Verification items for the finished model (mm, model axes). A direction names the side the tool comes from. Round coordinates to 2 decimals unless told otherwise and drop trailing zeros. Write each loop counter-clockwise with the first axis right and the second up, starting at its lowest first coordinate (ties: lowest second). Pieces come first, ordered by that corner, then holes. Notation, with made-up numbers: (82.25, 44) - (98.25, 44) arc R23 cw to (98.25, 55) - close; hole circle Ø1 at (23, 61.25). An arc over 180 degrees is marked (long way). Answer as a JSON object with one key per item and string values.
```python
from build123d import *

# Parameters (mm, degrees)
F1_R     = 22.710134
F2_DEPTH = 25


with BuildPart() as f2:
    # F1 (on Top) → F2 (new body)
    with BuildSketch(Plane.XY):
        with BuildLine():
            Line((3.498161, 48.480518), (0, 48.958581))
            Line((0, 48.958581), (-3.498161, 48.480518))
            Line((-3.498161, 48.480518), (-5.9562, 36.306892))
            ThreePointArc((-5.9562, 36.306892), (-11.369418, 34.991471), (-16.521988, 32.873859))
            Line((-16.521988, 32.873859), (-25.666062, 41.277731))
            Line((-25.666062, 41.277731), (-28.777132, 39.608324))
            Line((-28.777132, 39.608324), (-31.326205, 37.165396))
            Line((-31.326205, 37.165396), (-26.159323, 25.871926))
            ThreePointArc((-26.159323, 25.871926), (-29.765523, 21.625918), (-32.689339, 16.88413))
            Line((-32.689339, 16.88413), (-45.026722, 18.308253))
            Line((-45.026722, 18.308253), (-46.562377, 15.129034))
            Line((-46.562377, 15.129034), (-47.188704, 11.654355))
            Line((-47.188704, 11.654355), (-36.370473, 5.554763))
            ThreePointArc((-36.370473, 5.554763), (-36.79221, 0), (-36.370473, -5.554763))
            Line((-36.370473, -5.554763), (-47.188704, -11.654355))
            Line((-47.188704, -11.654355), (-46.562377, -15.129034))
            Line((-46.562377, -15.129034), (-45.026722, -18.308253))
            Line((-45.026722, -18.308253), (-32.689339, -16.88413))
            ThreePointArc((-32.689339, -16.88413), (-29.765523, -21.625918), (-26.159323, -25.871926))
            Line((-26.159323, -25.871926), (-31.326205, -37.165396))
            Line((-31.326205, -37.165396), (-28.777132, -39.608324))
            Line((-28.777132, -39.608324), (-25.666062, -41.277731))
            Line((-25.666062, -41.277731), (-16.521988, -32.873859))
            ThreePointArc((-16.521988, -32.873859), (-11.369418, -34.991471), (-5.9562, -36.306892))
            Line((-5.9562, -36.306892), (-3.498161, -48.480518))
            Line((-3.498161, -48.480518), (0, -48.958581))
            Line((0, -48.958581), (3.498161, -48.480518))
            Line((3.498161, -48.480518), (5.9562, -36.306892))
            ThreePointArc((5.9562, -36.306892), (11.369418, -34.991471), (16.521988, -32.873859))
            Line((16.521988, -32.873859), (25.666062, -41.277731))
            Line((25.666062, -41.277731), (28.777132, -39.608324))
            Line((28.777132, -39.608324), (31.326205, -37.165396))
            Line((31.326205, -37.165396), (26.159323, -25.871926))
            ThreePointArc((26.159323, -25.871926), (29.765523, -21.625918), (32.689339, -16.88413))
            Line((32.689339, -16.88413), (45.026722, -18.308253))
            Line((45.026722, -18.308253), (46.562377, -15.129034))
            Line((46.562377, -15.129034), (47.188704, -11.654355))
            Line((47.188704, -11.654355), (36.370473, -5.554763))
            ThreePointArc((36.370473, -5.554763), (36.79221, 0), (36.370473, 5.554763))
            Line((36.370473, 5.554763), (47.188704, 11.654355))
            Line((47.188704, 11.654355), (46.562377, 15.129034))
            Line((46.562377, 15.129034), (45.026722, 18.308253))
            Line((45.026722, 18.308253), (32.689339, 16.88413))
            ThreePointArc((32.689339, 16.88413), (29.765523, 21.625918), (26.159323, 25.871926))
            Line((26.159323, 25.871926), (31.326205, 37.165396))
            Line((31.326205, 37.165396), (28.777132, 39.608324))
            Line((28.777132, 39.608324), (25.666062, 41.277731))
            Line((25.666062, 41.277731), (16.521988, 32.873859))
            ThreePointArc((16.521988, 32.873859), (11.369418, 34.991471), (5.9562, 36.306892))
            Line((5.9562, 36.306892), (3.498161, 48.480518))
        make_face()
        Circle(F1_R, mode=Mode.SUBTRACT)
    extrude(amount=F2_DEPTH)


solid = f2.part
```
1. Cross-section at B-B (x = 15). Record the boundary of the cut face in (y, z), plus the area to 3 significant figures.
Completed:
{"outline": "(-33.6, 0) - (-17.05, 0) - (-17.05, 25) - (-33.6, 25) - close; (17.05, 0) - (33.6, 0) - (33.6, 25) - (17.05, 25) - close", "area": "827 mm^2"}
2. Go/stop test with flat-tipped pins: pin 1 (1 mm diameter, centred on x = 37, z = 16, fed in from -Y); pin 2 (1 mm diameter, centred on x = -7, y = 25, fed in from -Z); pin 3 (10 mm diameter, centred on x = -13.5, z = 4, fed in from -Y); pin 4 (4 mm diameter, centred on y = 24, z = 6, fed in from +X). Record where each tip stops, or that it passes through.
Completed:
{"pin 1": "stops at y = -17.44", "pin 2": "stops at z = 0", "pin 3": "stops at y = -35.8", "pin 4": "stops at x = 29.49"}
3. Cross-section at C-C (y = 28.5). Record the boundary of the cut face in (x, z), plus the area to 3 significant figures.
Completed:
{"outline": "(-27.36, 0) - (27.36, 0) - (27.36, 25) - (-27.36, 25) - close", "area": "1,370 mm^2"}
4. Cross-section at A-A (y = 0). Record the boundary of the cut face in (x, z), plus the area to 3 significant figures.
Completed:
{"outline": "(-36.79, 0) - (-22.71, 0) - (-22.71, 25) - (-36.79, 25) - close; (22.71, 0) - (36.79, 0) - (36.79, 25) - (22.71, 25) - close", "area": "704 mm^2"}
5. Mould release check, pull along X, two halves, no side actions. Record for faces 1 (the face through (-46.88, -13.37, 12.32)), 2 (the face through (11.295, -35.016, 12.325)), 3 (the face through (20, 12, 25)), 4 (the face through (-38.9, -17.6, 12.3)): released by +X, released by -X, zero draft, split by the parting line, or undercut.
Completed:
{"face 1": "released by -X", "face 2": "undercut", "face 3": "zero draft", "face 4": "undercut"}
6. Material ranges on probe 1 along Y at (x, z) = (0, 17); probe 2 along X at (y, z) = (36.5, 1.75); probe 3 along X at (y, z) = (-2, 18.5), recorded low to high. Write a range as from..to.
Completed:
{"probe 1": "y = -48.96..-22.71, 22.71..48.96", "probe 2": "x = -31.02..-20.47, -5.92..5.92, 20.47..31.02", "probe 3": "x = -36.74..-22.62, 22.62..36.74"}
7. Access from +Z, -Z, +X, -X, +Y, -Y to the whole of each face (thin tool, end or side, straight path). Record for faces 5 (the face through (-38.772, 17.586, 12.325)), 6 (the face through (4.71, -42.48, 12.32)), 7 (the face through (-28.78, 31.6, 12.32)).
Completed:
{"face 5": "+Z, -Z, +Y", "face 6": "+Z, -Z, -Y", "face 7": "+Z, -Z, -X"}
